Verification items for the finished model (mm, model axes). A direction names the side the tool comes from. Give positions to 0.01 mm unless a question says otherwise; leave off trailing zeros. Order: outer loops, then holes, each group sorted by start corner. A loop starts at its lowest first (then second) coordinate and runs counter-clockwise, first axis right, second up. Notation, with made-up numbers: M 43,-38.5 L 53,-38.5 A16 ccw 53,-17.5 Z; hole C 25.5,1 d10. An arc over 180 degrees is marked long. Answer as a JSON object with one key per item and string values.
```python
from build123d import *

# Parameters (mm, degrees)
F1_DEPTH    = 50.8
F2_W        = 38.1
F2_H        = 76.2
F3_DEPTH    = 25.4
F5_DEPTH    = 25.4
F6_T1_DEPTH = 6.35
F6_T3_DEPTH = 6.35


# Not quite as in the source:
# - a fillet or chamfer that OpenCascade refuses, or shapes differently, is made with other operations: its cross-section is extruded or revolved along the edge and cut away or added


with BuildPart() as f1:
    # F0 (on Right) → F1 (new body)
    with BuildSketch(Plane.YZ):
        Polygon((36.5886149989, -22.4861702016), (-39.6113850011, -22.4861702016), (-39.6113850011, -9.7861702016), (-45.9613837302, -9.7861702016), (-45.9613837302, -28.8361689307), (44.1562487973, -28.8361689307), (24.927321739, 80.2164955059), (18.673793759, 79.1138297984), align=None)
    extrude(amount=F1_DEPTH)

    # F2 (on face) → F3 (cut)
    with BuildSketch(Plane.XY.offset(-22.4861702016)):
        with Locations((25.4, -1.5113850011)):
            Rectangle(F2_W, F2_H)
    extrude(amount=-F3_DEPTH, mode=Mode.SUBTRACT)

    # F4 (on face) → F5 (cut)
    with BuildSketch(Plane(origin=(0, 37.8934996616, 6.6816463838), x_dir=(-1, 0, 0), z_dir=(0, 0.984807753, 0.1736481777))):
        Polygon((-25.4, 68.3192426996), (-44.45, -36.0657348664), (-6.35, -36.0657348664), align=None)
    extrude(amount=-F5_DEPTH, mode=Mode.SUBTRACT)

    # F6: chamfer of 6.35 on 4 edges, made by hand

    # F6_s2 → F6_t1 (join)
    with BuildSketch(Plane.YZ):
        Polygon((35.4859490708, -16.23264097), (30.2386149989, -22.4861702016), (36.5886149989, -22.4861702016), align=None)
    extrude(amount=F6_T1_DEPTH)

    # F6_s4 → F6_t3 (join)
    with BuildSketch(Plane.YZ.offset(44.45)):
        Polygon((35.4859490708, -16.23264097), (30.2386149989, -22.4861702016), (36.5886149989, -22.4861702016), align=None)
    extrude(amount=F6_T3_DEPTH)


solid = f1.part
```
Q1. Section check A-A on y = -21. Record the cut outline in (x, z).
Resolved:
{"outline": "M 0,-28.84 L 6.35,-28.84 L 6.35,-22.49 L 0,-22.49 Z; M 44.45,-28.84 L 50.8,-28.84 L 50.8,-22.49 L 44.45,-22.49 Z"}
Q2. Material ranges on L1, parallel to Y at x = 19, z = -14; L2, parallel to X at y = 23, z = 64; L3, parallel to Z at x = 29.5, y = -41, recorded low to high.
Resolved:
{"L1": "y = -45.96 to -39.61", "L2": "x = 0 to 23.71, 27.09 to 50.8", "L3": "z = -28.84 to -9.79"}
Q3. Section check C-C on z = -19. Record the cut outline in (x, y), then the cut area to 3 significant figures.
Resolved:
{"outline": "M 0,-45.96 L 50.8,-45.96 L 50.8,-39.61 L 0,-39.61 Z; M 0,33.16 L 6.35,33.16 L 6.35,35.97 L 8.38,35.97 L 8.17,42.42 L 0,42.42 Z; M 42.42,35.97 L 44.45,35.97 L 44.45,33.16 L 50.8,33.16 L 50.8,42.42 L 42.63,42.42 Z", "area": "465 mm²"}
Q4. Tool access check on faces 1 (the face through (25, -39.611, -19)), 2 (the face through (48, -4, -22.486)), 3 (the face through (6.35, -2, -25)). Record the directions out of +Z, -Z, +X, -X, +Y, -Y that give a thin tool (end or side, any length) a straight path to the whole face; none if there is none.
Resolved:
{"face 1": "+Z", "face 2": "+X, -X", "face 3": "-Z"}
Q5. Section check B-B on x = 35.5. Record the cut outline in (y, z), then the cut area to 3 significant figures.
Resolved:
{"outline": "M -45.96,-28.84 L -39.61,-28.84 L -39.61,-9.79 L -45.96,-9.79 Z; M 18.67,79.11 L 29.39,18.36 L 35.64,19.46 L 24.93,80.22 Z", "area": "513 mm²"}
Q6. Release check for a two-part mould opening along Y. For faces 4 (the face through (47.581, 32.899, -19.316)), 5 (the face through (13.76, 32.54, 37.04)), 6 (the face through (25.044, 21.844, 79.673)) record: +Y half, -Y half, draft (parallel to the pull), parting line (faces both ways), or undercut.
Resolved:
{"face 4": "undercut", "face 5": "+Y half", "face 6": "-Y half"}
Q7. Gauge pin test, flat ends, axial feed: pin 1 Ø21 at (x, z) = (14.5, -16) entering from +Y; pin 2 Ø3 at (x, y) = (45.5, -9) entering from +Z; pin 3 Ø6 at (x, z) = (30, 30.5) entering from -Y; pin 4 Ø3 at (x, y) = (23.5, -43) entering from +Z. Record the tip position at first contact, or that the pin passes through.
Resolved:
{"pin 1": "stops at y = 43.24", "pin 2": "stops at z = -22.49", "pin 3": "passes through", "pin 4": "stops at z = -9.79"}
Q8. Section check D-D on y = 23.5. Record the cut outline in (x, z).
Resolved:
{"outline": "M 0,-28.84 L 6.35,-28.84 L 6.35,-22.49 L 0,-22.49 Z; M 0,51.74 L 21.49,51.74 L 25.4,73.52 L 29.31,51.74 L 50.8,51.74 L 50.8,79.96 L 0,79.96 Z; M 44.45,-28.84 L 50.8,-28.84 L 50.8,-22.49 L 44.45,-22.49 Z"}
